Verification items for the finished model (mm, model axes). A direction names the side the tool comes from. Coordinates: 2 decimals unless noted, no trailing zeros. Write each loop counter-clockwise with the first axis right and the second up, starting at its lowest first coordinate (ties: lowest second). Pieces come first, ordered by that corner, then holes.
Autodesk Inventor part; units mm, degrees
ref_plane "YZ Plane" through (0, 0, 0) normal (1, 0, 0) x (0, 1, 0)
ref_plane "XZ Plane" through (0, 0, 0) normal (0, 1, 0) x (-1, 0, 0)
ref_plane "XY Plane" through (0, 0, 0) normal (0, 0, 1) x (1, 0, 0)
sketch "Skizze1" plane through (0, 0, 0) normal (0, 0, 1) x (1, 0, 0)
  circle A0 centre (0, 0) radius 29 construction
  circle A1 centre (0, 0) radius 33.5
  circle A2 centre (0, 0) radius 7.6
  circle A3 centre (0, 0) radius 9.6
  circle A4 centre (0, 0) radius 6.6
  line L0 (0, 46.9) -> (0, -46.9) construction
  line L1 (-46.9, 0) -> (46.9, 0) construction
  line L2 (-2, 25.923) -> (-2, 11.4263)
  line L3 (0, 0) -> (-28.9685, 16.725) construction
  line L4 (-23.4499, -11.2294) -> (-10.8955, -3.9811)
  arc A5 (-2, 11.4263) -> (-10.8955, -3.9811) centre (0, 0) ccw
  arc A6 (-2, 25.923) -> (-23.4499, -11.2294) centre (0, 0) ccw
  line L5 (21.4499, -14.6935) -> (8.8955, -7.4452)
  arc A7 (-21.4499, -14.6935) -> (21.4499, -14.6935) centre (0, 0) ccw
  line L6 (-21.4499, -14.6935) -> (-8.8955, -7.4452)
  arc A8 (-8.8955, -7.4452) -> (8.8955, -7.4452) centre (0, 0) ccw
  line L7 (2, 25.923) -> (2, 11.4263)
  arc A9 (23.4499, -11.2294) -> (2, 25.923) centre (0, 0) ccw
  line L8 (23.4499, -11.2294) -> (10.8955, -3.9811)
  arc A10 (10.8955, -3.9811) -> (2, 11.4263) centre (0, 0) ccw
  circle A11 centre (0, 29) radius 2.1
  circle A12 centre (-14.5, 25.1147) radius 2.1
  circle A13 centre (-25.1147, 14.5) radius 2.1
  circle A14 centre (-29, 0) radius 2.1
  circle A15 centre (-25.1147, -14.5) radius 2.1
  circle A16 centre (-14.5, -25.1147) radius 2.1
  circle A17 centre (0, -29) radius 2.1
  circle A18 centre (14.5, -25.1147) radius 2.1
  circle A19 centre (25.1147, -14.5) radius 2.1
  circle A20 centre (29, 0) radius 2.1
  circle A21 centre (25.1147, 14.5) radius 2.1
  circle A22 centre (0, 0) radius 31.9
  circle A23 centre (14.5, 25.1147) radius 2.1
  dimension "d1" = 29
  dimension "d2" = 15.2
  dimension "d3" = 2
  dimension "d12" = 1
  dimension "d17" = 60
  dimension "d18" = 2
  dimension "d19" = 3
  dimension "d20" = 2
  dimension "d23" = 360
  dimension "d28" = 4.2
  dimension "d31" = 360
  dimension "d33" = 63.8
  dimension "d35" = 67
extrude "Extrusion1" add sketch "Skizze1" along normal blind 2 contours A1 | A3 | A11 | A12 | A13 | A14 | A15 | A16 | A17 | A18 | A19 | A20 | A21 | A22 | A23
extrude "Extrusion2" add sketch "Skizze1" along normal blind 2 from surface at 2 contours A3 | A22
extrude "Extrusion3" add sketch "Skizze1" against normal blind 3 from surface at 0 contours A3
extrude "Extrusion4" add sketch "Skizze1" against normal blind 1.5 from surface at -3 contours A2 | A3
properties part number "ShaftHolder2"
1. Sectioned sample at C-C, the plane y = 18. Record the boundary of the cut face in (x, z).
2. Draft check along Y on faces 1 (the flat face through (-7, -2, -4.5)), 2 (the cylindrical face through (-13.371, 23.344, 2.986)). Enter one of: pulls with the +Y half, pulls with the -Y half, needs draft (parallel to the pull), parting line crosses it, or undercut.
3. Material ranges on L1, parallel to Y at x = 0, z = 0.25; L2, parallel to X at y = -26.5, z = 2.25; L3, parallel to Y at x = -3, z = 2.5, recorded low to high.
4. Sectioned sample at D-D, the plane x = 29. Record the boundary of the cut face in (y, z), and give its area (3 significant figures).
5. Sectioned sample at A-A, the plane x = 0. Give the number of separate pieces and of enclosed holes in the cut face, and give its area (3 significant figures).
6. Tool access check on faces 3 (the flat face through (15.26, -11.12, 1.97)), 4 (the flat face through (14, -25, 2)). Record the directions out of +Z, -Z, +X, -X, +Y, -Y that give a thin tool (end or side, any length) a straight path to the whole face; none if there is none.
7. Gauge pin test, flat ends, axial feed: P1, Ø5, axis at x = -25.11, y = 14.5, coming from the -Z side; P2, Ø2.5, axis at x = 25.11, y = 14.5, coming from the +Z side; P3, Ø3, axis at y = 19, z = 3, coming from the -X side. Record the tip position at first contact, or that the pin passes through.
8. Sectioned sample at B-B, the plane z = 1. Record the boundary of the cut face in (x, y), and give its area (3 significant figures).
Outcome:
1. outline: (-28.25, 0) - (-18.76, 0) - (-18.76, 4) - (-26.34, 4) - (-26.34, 2) - (-28.25, 2) - close; (-2, 0) - (2, 0) - (2, 4) - (-2, 4) - close; (18.76, 0) - (28.25, 0) - (28.25, 2) - (26.34, 2) - (26.34, 4) - (18.76, 4) - close
2. face 1: needs draft
2. face 2: undercut
3. L1: y = -33.5 to -26, -11.6 to -7.6, 7.6 to 33.5
3. L2: x = -17.76 to -16.08, -12.92 to 12.92, 16.08 to 17.76
3. L3: y = -31.76 to -25.83, -11.21 to -6.98, 6.98 to 11.21, 25.83 to 31.76
4. outline: (-16.77, 0) - (16.77, 0) - (16.77, 2) - (13.29, 2) - (13.29, 4) - (2.1, 4) - (2.1, 2) - (-2.1, 2) - (-2.1, 4) - (-13.29, 4) - (-13.29, 2) - (-16.77, 2) - close
4. area: 112 mm2
5. separate pieces: 3
5. enclosed holes: 0
5. area: 147 mm2
6. face 3: +Z, -Z
6. face 4: +Z
7. P1: stops at z = 0
7. P2: stops at z = 2
7. P3: stops at x = -28.33
8. outline: circle Ø67 at (0, 0); hole (-23.45, -11.23) - (-10.9, -3.98) arc R11.6 cw to (-2, 11.43) - (-2, 25.92) arc R26 ccw to start; hole (-21.45, -14.69) arc R26 ccw to (21.45, -14.69) - (8.9, -7.45) arc R11.6 cw to (-8.9, -7.45) - close; hole circle Ø15.2 at (0, 0); hole (2, 11.43) arc R11.6 cw to (10.9, -3.98) - (23.45, -11.23) arc R26 ccw to (2, 25.92) - close
8. area: 1,820 mm2
